```python
from build123d import *

# Parameters (mm, degrees)
SKETCH1_W           = 114.3
SKETCH1_H           = 31.75
SKETCH1_R           = 0.9115
SKETCH1_R_2         = 4
SKETCH1_R_3         = 1.7
BOSS_EXTRUDE1_DEPTH = 6.35


with BuildPart() as part:
    # Sketch1 → Boss-Extrude1 (new body)
    with BuildSketch(Plane.XY):
        Rectangle(SKETCH1_W, SKETCH1_H)
        with Locations((-9.000000134, 0)):
            Circle(SKETCH1_R, mode=Mode.SUBTRACT)
        with Locations((0, -9.000000134)):
            Circle(SKETCH1_R, mode=Mode.SUBTRACT)
        with Locations((9.000000134, 0)):
            Circle(SKETCH1_R, mode=Mode.SUBTRACT)
        with Locations((0, 9.000000134)):
            Circle(SKETCH1_R, mode=Mode.SUBTRACT)
        with Locations((-43.000000106, 0)):
            Circle(SKETCH1_R_2, mode=Mode.SUBTRACT)
        with Locations((43.000000106, 0)):
            Circle(SKETCH1_R_2, mode=Mode.SUBTRACT)
        with Locations((-36.264808015, 6.735192091)):
            Circle(SKETCH1_R_3, mode=Mode.SUBTRACT)
        with Locations((-49.735192197, 6.735192091)):
            Circle(SKETCH1_R_3, mode=Mode.SUBTRACT)
        with Locations((-36.264808015, -6.735192091)):
            Circle(SKETCH1_R_3, mode=Mode.SUBTRACT)
        with Locations((-49.735192197, -6.735192091)):
            Circle(SKETCH1_R_3, mode=Mode.SUBTRACT)
        with Locations((49.735192197, -6.735192091)):
            Circle(SKETCH1_R_3, mode=Mode.SUBTRACT)
        with Locations((36.264808015, -6.735192091)):
            Circle(SKETCH1_R_3, mode=Mode.SUBTRACT)
        with Locations((36.264808015, 6.735192091)):
            Circle(SKETCH1_R_3, mode=Mode.SUBTRACT)
        with Locations((49.735192197, 6.735192091)):
            Circle(SKETCH1_R_3, mode=Mode.SUBTRACT)
        with BuildLine():
            Line((-6.79791666, -1.758075393), (-1.758075393, -6.79791666))
            ThreePointArc((-1.758075393, -6.79791666), (-1.714608205, -6.830865544), (-1.663855614, -6.850845531))
            ThreePointArc((-1.663855614, -6.850845531), (4.985102807, -4.985102807), (6.850845531, 1.663855614))
            ThreePointArc((6.850845531, 1.663855614), (6.830865544, 1.714608205), (6.79791666, 1.758075393))
            Line((6.79791666, 1.758075393), (1.758075393, 6.79791666))
            ThreePointArc((1.758075393, 6.79791666), (1.714608205, 6.830865544), (1.663855614, 6.850845531))
            ThreePointArc((1.663855614, 6.850845531), (-4.985102807, 4.985102807), (-6.850845531, -1.663855614))
            ThreePointArc((-6.850845531, -1.663855614), (-6.830865544, -1.714608205), (-6.79791666, -1.758075393))
        make_face(mode=Mode.SUBTRACT)
    extrude(amount=BOSS_EXTRUDE1_DEPTH)


solid = part.part
```
The listing builds one solid part. Answer for the finished solid, in the listing's coordinates (mm). A direction names the side the tool comes from. Round coordinates to 2 decimals unless told otherwise and drop trailing zeros. Order: outer loops, then holes, each group sorted by start corner. A loop starts at its lowest first (then second) coordinate and runs counter-clockwise, first axis right, second up. Notation, with made-up numbers: (14.5, 32.25) -> (57.5, 32.25) arc R5 cw to (57.5, 38.25) -> close; hole circle Ø2 at (37, -19). An arc over 180 degrees is marked (long way). Answer as CSV lines item,"result". Start each with the question number.
(1) The part is cut by section A-A (x = -43). Determine the outline of the cut face in (y, z) (3 decimals).
(2) Find the intervals of material crossed by probe 1 along X at (y, z) = (-0.5, 5); probe 2 along Y at (x, z) = (-9, 4.5) (1 decimal); probe 3 along X at (y, z) = (7.5, 1.75), in increasing order. Write a range as from..to.
(3) A flat-ended cylindrical pin translates along its axis: pin 1 Ø7 at (x, y) = (-43, 0) entering from -Z. Find the tip coordinate at first contact, or state that the pin passes through.
(4) The part is cut by section B-B (z = 2.25). Count the separate pieces of the cut face and the enclosed holes in it, then the cut area to 3 significant figures.
(5) For a pull along Y with two mould halves and no side action, classify faces 3 (the face through (-0.8, 7.3, 0)), 4 (the face through (-1, -15.875, 3)), 5 (the face through (-1, 15.875, 3)), 6 (the face through (-39.185, 1.201, 3.131)) as +Y half, -Y half, draft (parallel to the pull), parting line (faces both ways), or undercut.
(6) A tool of negligible diameter and unlimited length cuts with its end or side. For faces 1 (the face through (4.313, 4.243, 3.131)), 2 (the face through (-57.15, 0, 3)), from which of +Z, -Z, +X, -X, +Y, -Y can it reach the whole face along a straight path? Write none if from no direction.
Evaluation:
1,outline,"(-15.875, 0) -> (-4, 0) -> (-4, 6.35) -> (-15.875, 6.35) -> close; (4, 0) -> (15.875, 0) -> (15.875, 6.35) -> (4, 6.35) -> close"
2,probe 1,"-57.15..-46.97, -39.03..-9.76, -8.24..-7.03, 7.03..8.24, 9.76..39.03, 46.97..57.15"
2,probe 2,"-15.9..-0.9, 0.9..15.9"
2,probe 3,"-57.15..-51.25, -48.22..-37.78, -34.75..34.75, 37.78..48.22, 51.25..57.15"
3,pin 1,"through"
4,separate pieces,"1"
4,enclosed holes,"15"
4,area,"3,300 mm²"
5,face 3,"draft"
5,face 4,"-Y half"
5,face 5,"+Y half"
5,face 6,"undercut"
6,face 1,"+Z, -Z"
6,face 2,"+Z, -Z, -X, +Y, -Y"
